Can you work these out from the drawing? Everything is in mm from the part's minimum corner. Round coordinates to 2 decimals unless told otherwise and drop trailing zeros. Loops run counter-clockwise (first coordinate to the right, second up) from the corner with the lowest first, then second, coordinate; pieces in that order, holes last. Notation, with made-up numbers: (-18.75, 39) -> (-4.75, 39) arc R6 ccw to (-4.75, 45) -> close; hole circle Ø5 at (-22.75, 32.25). An arc over 180 degrees is marked (long way). One line per item, written item: value.
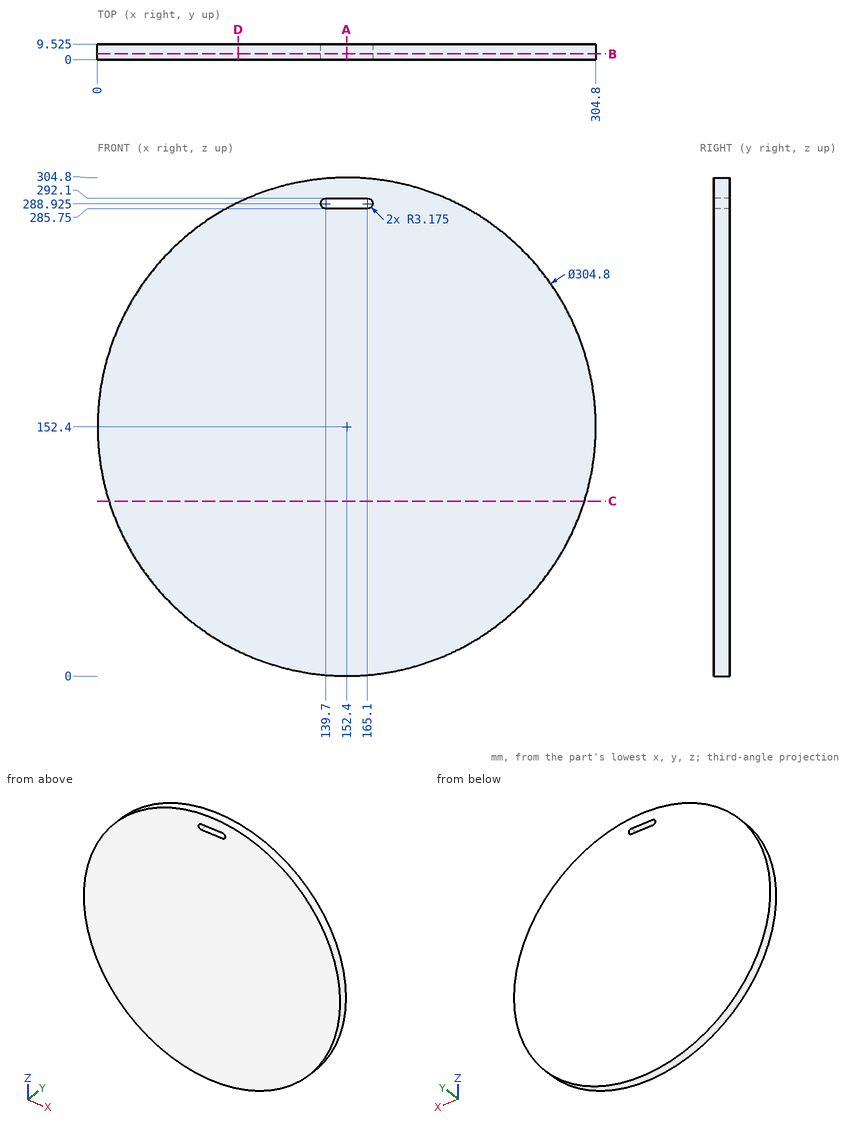
(1) I'm going to push flat-ended pins straight in: pin 1 Ø5 at (x, y) = (79, 5) entering from +Z; pin 2 Ø1 at (y, z) = (7, 189.5) entering from +X; pin 3 Ø1.5 at (x, y) = (128, 3.5) entering from -Z. Where does each tip first touch, or does it pass through?
Recorded:
pin 1: z = 287.3
pin 2: x = 300.34
pin 3: z = 1.85
(2) If we section it at A-A, the plane x = 152.4: Please give me the cut outline in (y, z) (3 decimals), then the cut area to 3 significant figures.
Recorded:
outline: (0, 0) -> (9.525, 0) -> (9.525, 285.75) -> (0, 285.75) -> close; (0, 292.1) -> (9.525, 292.1) -> (9.525, 304.8) -> (0, 304.8) -> close
area: 2,840 mm²
(3) If we section it at B-B, the plane y = 3.5: Please give me the cut outline in (x, z) (3 decimals).
Recorded:
outline: circle Ø304.8 at (152.4, 152.4); hole (139.7, 285.75) -> (165.1, 285.75) arc R3.175 ccw to (165.1, 292.1) -> (139.7, 292.1) arc R3.175 ccw to start
(4) If I drill on L1, parallel to Z at x = 144.5, y = 6; L2, parallel to X at y = 4, z = 156.5; L3, parallel to Z at x = 147.5, y = 6.25, over which ranges is the centre line in solid material (lowest first)?
Recorded:
L1: 0.2 to 285.75, 292.1 to 304.6
L2: 0.06 to 304.74
L3: 0.08 to 285.75, 292.1 to 304.72
(5) If we section it at D-D, the plane x = 86: Please give me the cut outline in (y, z) (3 decimals).
Recorded:
outline: (0, 15.226) -> (9.525, 15.226) -> (9.525, 289.574) -> (0, 289.574) -> close
(6) If we section it at C-C, the plane z = 107: Please give me the cut outline in (x, y) (3 decimals).
Recorded:
outline: (6.919, 0) -> (297.881, 0) -> (297.881, 9.525) -> (6.919, 9.525) -> close
